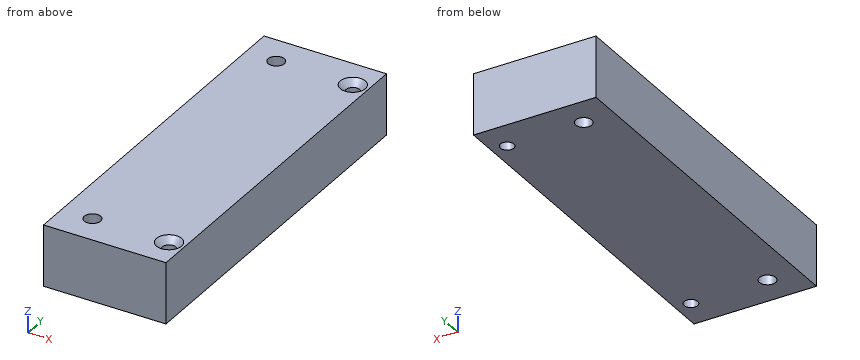
```python
from build123d import *

# Parameters (mm, degrees)
SKETCH1_W                                          = 50.8
SKETCH1_H                                          = 152.4
SKETCH1_R                                          = 3.3782
BOSS_EXTRUDE1_DEPTH                                = 25.4
CSK_FOR_10_FLAT_HEAD_SOCKET_CAP_SCREW1_D           = 5.6134
CSK_FOR_10_FLAT_HEAD_SOCKET_CAP_SCREW1_CSINK_D     = 10.4394
CSK_FOR_10_FLAT_HEAD_SOCKET_CAP_SCREW1_CSINK_ANGLE = 82


with BuildPart() as part:
    # Sketch1 → Boss-Extrude1 (new body)
    with BuildSketch(Plane.XY):
        with Locations((330.2, 241.3)):
            Rectangle(SKETCH1_W, SKETCH1_H)
        with Locations((317.5, 304.8)):
            Circle(SKETCH1_R, mode=Mode.SUBTRACT)
        with Locations((317.5, 177.8)):
            Circle(SKETCH1_R, mode=Mode.SUBTRACT)
    extrude(amount=BOSS_EXTRUDE1_DEPTH)

    # CSK for #10 Flat Head Socket Cap Screw1 (through all)
    with Locations(Plane.XY.offset(25.4)):
        with Locations((349.25, 304.8), (349.25, 177.8)):
            CounterSinkHole(CSK_FOR_10_FLAT_HEAD_SOCKET_CAP_SCREW1_D / 2, CSK_FOR_10_FLAT_HEAD_SOCKET_CAP_SCREW1_CSINK_D / 2, counter_sink_angle=CSK_FOR_10_FLAT_HEAD_SOCKET_CAP_SCREW1_CSINK_ANGLE)


solid = part.part
```
CAD build for the part. Positions are in the model's coordinates, mm. Coordinates: 2 decimals unless noted, no trailing zeros. Order: outer loops, then holes, each group sorted by start corner. A loop starts at its lowest first (then second) coordinate and runs counter-clockwise, first axis right, second up. Notation, with made-up numbers: (-19.75, -20) - (7.25, -20) arc R25 ccw to (7.25, -1) - close; hole circle Ø11 at (18, -12). An arc over 180 degrees is marked (long way). Answer in a Markdown table with one row per item.
1. Slice it at D-D, the plane x = 319.5. List the corners of the cut face in (y, z), then the cut area to 3 significant figures.
Answer:
| item | result |
|---|---|
| outline | (165.1, 0) - (175.08, 0) - (175.08, 25.4) - (165.1, 25.4) - close; (180.52, 0) - (302.08, 0) - (302.08, 25.4) - (180.52, 25.4) - close; (307.52, 0) - (317.5, 0) - (317.5, 25.4) - (307.52, 25.4) - close |
| area | 3,590 mm² |
2. Drill centre lines: L1, parallel to X at y = 177.8, z = 12.5; L2, parallel to Y at x = 317.5, z = 10.75; L3, parallel to Y at x = 349.25, z = 15. Where is each one in solid material? Low to high. Write a range as from..to.
Answer:
| item | result |
|---|---|
| L1 | 304.8..314.12, 320.88..346.44, 352.06..355.6 |
| L2 | 165.1..174.42, 181.18..301.42, 308.18..317.5 |
| L3 | 165.1..174.99, 180.61..301.99, 307.61..317.5 |
3. Slice it at A-A, the plane x = 349.25. List the corners of the cut face in (y, z), then the cut area to 3 significant figures.
Answer:
| item | result |
|---|---|
| outline | (165.1, 0) - (174.99, 0) - (174.99, 22.62) - (172.58, 25.4) - (165.1, 25.4) - close; (180.61, 0) - (301.99, 0) - (301.99, 22.62) - (299.58, 25.4) - (183.02, 25.4) - (180.61, 22.62) - close; (307.61, 0) - (317.5, 0) - (317.5, 25.4) - (310.02, 25.4) - (307.61, 22.62) - close |
| area | 3,570 mm² |
4. Slice it at C-C, the plane z = 13.25. List the corners of the cut face in (x, y), then the cut area to 3 significant figures.
Answer:
| item | result |
|---|---|
| outline | (304.8, 165.1) - (355.6, 165.1) - (355.6, 317.5) - (304.8, 317.5) - close; hole circle Ø6.76 at (317.5, 177.8); hole circle Ø6.76 at (317.5, 304.8); hole circle Ø5.61 at (349.25, 177.8); hole circle Ø5.61 at (349.25, 304.8) |
| area | 7,620 mm² |
5. Slice it at B-B, the plane y = 304.8. List the corners of the cut face in (x, z), then the cut area to 3 significant figures.
Answer:
| item | result |
|---|---|
| outline | (304.8, 0) - (314.12, 0) - (314.12, 25.4) - (304.8, 25.4) - close; (320.88, 0) - (346.44, 0) - (346.44, 22.62) - (344.03, 25.4) - (320.88, 25.4) - close; (352.06, 0) - (355.6, 0) - (355.6, 25.4) - (354.47, 25.4) - (352.06, 22.62) - close |
| area | 969 mm² |
